Verification items for this drawing (mm, ordinates from the low corner). A direction names the side the tool comes from. Round coordinates to 2 decimals unless told otherwise and drop trailing zeros. Order: outer loops, then holes, each group sorted by start corner. A loop starts at its lowest first (then second) coordinate and runs counter-clockwise, first axis right, second up. Notation, with made-up numbers: (65, 10) -> (109, 10) arc R29 cw to (109, 38) -> close; hole circle Ø9 at (12.25, -38.5). An arc over 180 degrees is marked (long way). Return JSON: item names as keys, results as strings. Group by question number.
Item 1: Sectioned sample at C-C on x = 20. Record the cut outline in (y, z).
Item 2: Depth check by flat-ended pin: pin 1 Ø12 at (x, z) = (16.5, 22) entering from +Y; pin 2 Ø8 at (x, y) = (10.5, 34.5) entering from +Z; pin 3 Ø2 at (y, z) = (27, 25) entering from +X; pin 4 Ø5 at (x, y) = (7.5, 28.5) entering from -Z. Enter the tip coordinate at first touch or a pass-through.
Item 3: Sectioned sample at B-B on x = 25.5. Record the cut outline in (y, z), plus the area to 3 significant figures.
Item 4: Access from +Z, -Z, +X, -X, +Y, -Y to the whole of each face (thin tool, end or side, straight path). Record for the marked faces 1 and 2.
Item 5: Sectioned sample at A-A on z = 42.85. Record the cut outline in (x, y), plus the area to 3 significant figures.
Item 6: Scan lines: probe 1 along Z at (x, y) = (20, 12.5); probe 2 along X at (y, z) = (33, 12.5); probe 3 along X at (y, z) = (10, 24). Record each from-to range of solid material in increasing order. Write a range as from..to.
Item 7: Sectioned sample at D-D on y = 36.5. Record the cut outline in (x, z), plus the area to 3 significant figures.
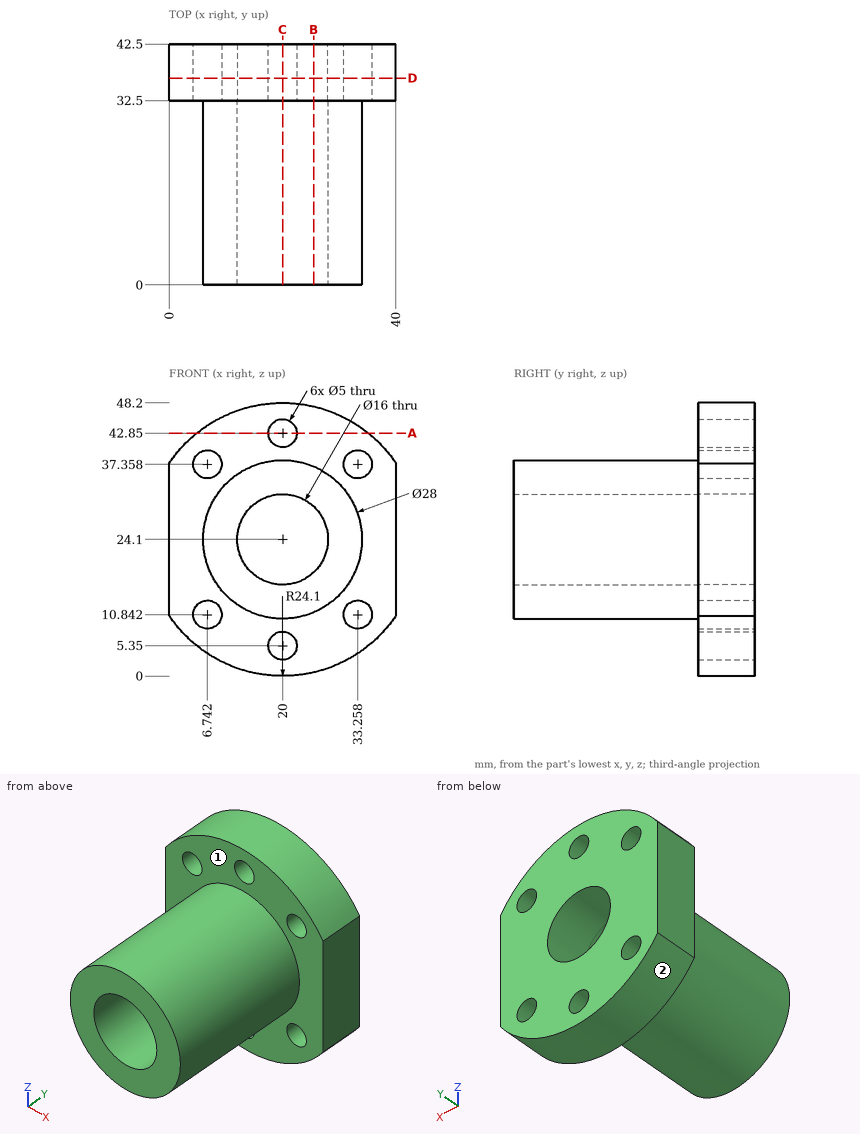
Recorded:
{
 "1": {"outline": "(0, 10.1) -> (32.5, 10.1) -> (32.5, 7.85) -> (42.5, 7.85) -> (42.5, 16.1) -> (0, 16.1) -> close; (0, 32.1) -> (42.5, 32.1) -> (42.5, 40.35) -> (32.5, 40.35) -> (32.5, 38.1) -> (0, 38.1) -> close; (32.5, 0) -> (42.5, 0) -> (42.5, 2.85) -> (32.5, 2.85) -> close; (32.5, 45.35) -> (42.5, 45.35) -> (42.5, 48.2) -> (32.5, 48.2) -> close"},
 "2": {"pin 1": "y = 42.5", "pin 2": "z = 47.56", "pin 3": "x = 34", "pin 4": "z = 14.3"},
 "3": {"outline": "(0, 11.23) -> (32.5, 11.23) -> (32.5, 0.64) -> (42.5, 0.64) -> (42.5, 18.29) -> (0, 18.29) -> close; (0, 29.91) -> (42.5, 29.91) -> (42.5, 47.56) -> (32.5, 47.56) -> (32.5, 36.97) -> (0, 36.97) -> close", "area": "812 mm²"},
 "4": {"face 1": "-Y", "face 2": "-Z, +Y, -Y"},
 "5": {"outline": "(4.86, 32.5) -> (17.5, 32.5) -> (17.5, 42.5) -> (4.86, 42.5) -> close; (22.5, 32.5) -> (35.14, 32.5) -> (35.14, 42.5) -> (22.5, 42.5) -> close", "area": "253 mm²"},
 "6": {"probe 1": "10.1..16.1, 32.1..38.1", "probe 2": "0..4.87, 8.61..31.39, 35.13..40", "probe 3": "6..12, 28..34"},
 "7": {"outline": "(0, 10.65) arc R24.1 ccw to (40, 10.65) -> (40, 37.55) arc R24.1 ccw to (0, 37.55) -> close; hole circle Ø5 at (6.74, 10.84); hole circle Ø5 at (6.74, 37.36); hole circle Ø16 at (20, 24.1); hole circle Ø5 at (20, 5.35); hole circle Ø5 at (20, 42.85); hole circle Ø5 at (33.26, 10.84); hole circle Ø5 at (33.26, 37.36)", "area": "1,360 mm²"}
}
